from build123d import *

# Parameters (mm, degrees)
SM_BASE_FLANGE_1_DEPTH = 543
SKETCH_7_R             = 3.5
CUT_EXTRUDE_2_DEPTH    = 10
SKETCH_8_R             = 6.5
CUT_EXTRUDE_3_DEPTH    = 10


# Sheet-metal steps are written as plain solids
with BuildPart() as part:
    # Sketch 1 → Базовая кромка1 (new, symmetric)
    with BuildSketch(Plane.XY):
        with BuildLine():
            Line((-71.75, -30.5), (-39.75, -30.5))
            ThreePointArc((-39.75, -30.5), (-37.628679656, -29.621320344), (-36.75, -27.5))
            Line((-36.75, -27.5), (-36.75, -1.5))
            ThreePointArc((-36.75, -1.5), (-36.310660172, -0.439339828), (-35.25, 0))
            Line((-35.25, 0), (35.25, 0))
            ThreePointArc((35.25, 0), (36.310660172, -0.439339828), (36.75, -1.5))
            Line((36.75, -1.5), (36.75, -27.5))
            ThreePointArc((36.75, -27.5), (37.628679656, -29.621320344), (39.75, -30.5))
            Line((39.75, -30.5), (71.75, -30.5))
            Line((71.75, -30.5), (71.75, -29))
            Line((71.75, -29), (39.75, -29))
            ThreePointArc((39.75, -29), (38.689339828, -28.560660172), (38.25, -27.5))
            Line((38.25, -27.5), (38.25, -1.5))
            ThreePointArc((38.25, -1.5), (37.371320344, 0.621320344), (35.25, 1.5))
            Line((35.25, 1.5), (-35.25, 1.5))
            ThreePointArc((-35.25, 1.5), (-37.371320344, 0.621320344), (-38.25, -1.5))
            Line((-38.25, -1.5), (-38.25, -27.5))
            ThreePointArc((-38.25, -27.5), (-38.689339828, -28.560660172), (-39.75, -29))
            Line((-39.75, -29), (-71.75, -29))
            Line((-71.75, -29), (-71.75, -30.5))
        make_face()
    extrude(amount=SM_BASE_FLANGE_1_DEPTH, both=True)

    # Эскиз7 → Вырез-Вытянуть2 (cut)
    with BuildSketch(Plane.XZ.offset(30.5)):
        with Locations((56.75, 528)):
            Circle(SKETCH_7_R)
        with Locations((-56.75, 528)):
            Circle(SKETCH_7_R)
        with Locations((56.75, -528)):
            Circle(SKETCH_7_R)
        with Locations((-56.75, -528)):
            Circle(SKETCH_7_R)
    extrude(amount=-CUT_EXTRUDE_2_DEPTH, mode=Mode.SUBTRACT)

    # Эскиз8 → Вырез-Вытянуть3 (cut)
    with BuildSketch(Plane(origin=(0, 1.5, 0), x_dir=(1, 0, 0), z_dir=(0, 1, 0))):
        with Locations(Location((0, 210, 0), (0, 0, 270))):
            Circle(SKETCH_8_R)
        with Locations(Location((0, 0, 0), (0, 0, 270))):
            Circle(SKETCH_8_R)
        with Locations(Location((0, -210, 0), (0, 0, 270))):
            Circle(SKETCH_8_R)
    extrude(amount=-CUT_EXTRUDE_3_DEPTH, mode=Mode.SUBTRACT)


solid = part.part
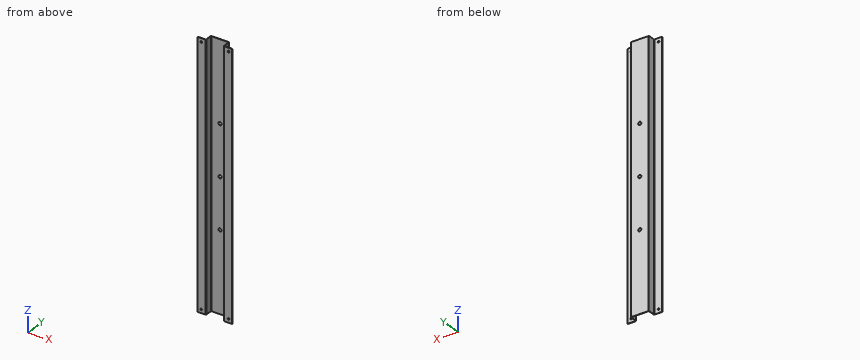
Read the model definition and answer for the solid it produces. Units are mm, in the model's axes. Round coordinates to 2 decimals unless told otherwise and drop trailing zeros. Write each loop counter-clockwise with the first axis right and the second up, starting at its lowest first coordinate (ties: lowest second). Pieces come first, ordered by that corner, then holes. Notation, with made-up numbers: M -13,-8.5 L 11,-8.5 A18 ccw 11,8.5 Z; hole C -25.75,14 d8. An arc over 180 degrees is marked long. Use a Markdown table: item, result.
1) The part is cut by section A-A (y = -21.5). Write down the section's boundary in (x, z).
Answers follow:
| item | result |
|---|---|
| outline | M -38.25,-543 L -36.75,-543 L -36.75,543 L -38.25,543 Z; M 36.75,-543 L 38.25,-543 L 38.25,543 L 36.75,543 Z |
2) The part is cut by section B-B (z = 62). Write down the section's boundary in (x, y), plus the area to 3 significant figures.
Answers follow:
| item | result |
|---|---|
| outline | M -71.75,-30.5 L -39.75,-30.5 A3 ccw -36.75,-27.5 L -36.75,-1.5 A1.5 cw -35.25,0 L 35.25,0 A1.5 cw 36.75,-1.5 L 36.75,-27.5 A3 ccw 39.75,-30.5 L 71.75,-30.5 L 71.75,-29 L 39.75,-29 A1.5 cw 38.25,-27.5 L 38.25,-1.5 A3 ccw 35.25,1.5 L -35.25,1.5 A3 ccw -38.25,-1.5 L -38.25,-27.5 A1.5 cw -39.75,-29 L -71.75,-29 Z |
| area | 301 mm2 |
3) Flat-ended cylindrical pins translate along their axes: pin 1 (2 mm diameter, centred on y = -27, z = 246, fed in from -X); pin 2 (9 mm diameter, centred on x = -56.75, z = -528, fed in from +Y); pin 3 (3 mm diameter, centred on y = -18.5, z = 434.5, fed in from +X); pin 4 (1.5 mm diameter, centred on x = 34.5, y = -15, fed in from +Z). Find the tip coordinate at first contact, or state that the pin passes through.
Answers follow:
| item | result |
|---|---|
| pin 1 | stops at x = -38.34 |
| pin 2 | stops at y = -29 |
| pin 3 | stops at x = 38.25 |
| pin 4 | passes through |
4) Straight lines are drawn through the part: line 1 along Z through (x, y) = (-56.75, -29.95); line 2 along X through (y, z) = (-8.5, -388.5); line 3 along X through (y, z) = (-29.75, -528). For each, find the intervals that lie inside material, in ascending order. Write a range as [from, to].
Answers follow:
| item | result |
|---|---|
| line 1 | z = [-543, -531.5], [-524.5, 524.5], [531.5, 543] |
| line 2 | x = [-38.25, -36.75], [36.75, 38.25] |
| line 3 | x = [-71.75, -60.25], [-53.25, -37.77], [37.77, 53.25], [60.25, 71.75] |
